```python
from build123d import *

# Parameters (mm, degrees)
F0_W     = 10
F0_H     = 25.0418604054
F0_H_2   = 18
F0_H_3   = 6.9581395946
F3_R     = 10
F4_DEPTH = 141.6
F7_D     = 3
F8_D     = 3
F9_R     = 2.99999


# Not quite as in the source:
# - a fillet or chamfer that OpenCascade refuses, or shapes differently, is made with other operations: its cross-section is extruded or revolved along the edge and cut away or added
# - a fillet or chamfer is up to 0.001 mm smaller than in the source, because OpenCascade refuses the exact size


with BuildPart() as f1:
    # F0 (on Front) → F1 (revolve)
    with BuildSketch(Plane.XZ):
        Polygon((-55, 15), (-55, 0), (0, 0), (0, 18), (-40, 18), (-40, 15), align=None)
    revolve(axis=Axis((0, 0, 9), (0, 0, 1)))

    # F0 (on Front) → F2 (revolve, cut)
    with BuildSketch(Plane.XZ):
        with Locations((5, 30.5209302027)):
            Rectangle(F0_W, F0_H)
        with Locations((5, 9)):
            Rectangle(F0_W, F0_H_2)
        with Locations((5, -3.4790697973)):
            Rectangle(F0_W, F0_H_3)
    revolve(axis=Axis((0, 0, 18.0418604054), (0, 0, 1)), mode=Mode.SUBTRACT)

    # F3 (on Front) → F4 (cut)
    with BuildSketch(Plane.XZ):
        Circle(F3_R)
    extrude(amount=-F4_DEPTH, mode=Mode.SUBTRACT)

    # F5: fillet of radius 15 on 1 edges, made by hand

    # F5_s1 → F5_t2 (revolve, cut)
    with BuildSketch(Plane.XZ):
        with BuildLine():
            ThreePointArc((-55, 0), (-50.6066017178, 10.6066017178), (-40, 15))
            Line((-40, 15), (-55, 15))
            Line((-55, 15), (-55, 0))
        make_face()
    revolve(axis=Axis((0, 0, 15), (0, 0, 1)), mode=Mode.SUBTRACT)

    # F7 (through all)
    with Locations(Plane(origin=(0, 0, 0), x_dir=(1, 0, 0), z_dir=(0, 0, -1))):
        with Locations((24, 0)):
            Hole(F7_D / 2)

    # F8 (through all)
    with Locations(Plane(origin=(0, 0, 0), x_dir=(1, 0, 0), z_dir=(0, 0, -1))):
        with Locations((-24, 0)):
            Hole(F8_D / 2)

    # F9 (radius 3 in the source; OpenCascade refuses exactly that, so slightly less here)
    f9_edges = [f1.edges().sort_by_distance(p)[0] for p in [
        (40, 0, 18),
    ]]
    fillet(f9_edges, radius=F9_R)


solid = f1.part
```
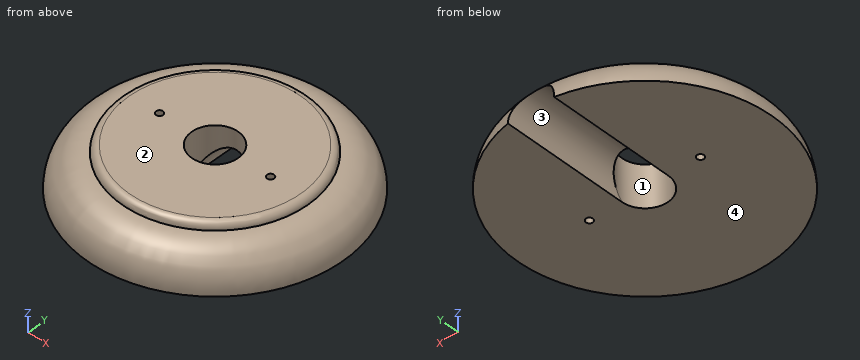
Here's how the part is built. I have some questions about the finished solid (model axes, mm). Face numbers are marked on the shaded views. A direction names the side the tool comes from. Coordinates: 2 decimals unless noted, no trailing zeros. Order: outer loops, then holes, each group sorted by start corner. A loop starts at its lowest first (then second) coordinate and runs counter-clockwise, first axis right, second up. Notation, with made-up numbers: (69, 79) - (89, 79) arc R36 cw to (89, 117) - close; hole circle Ø4 at (71.5, 55.5). An arc over 180 degrees is marked (long way). One line per question, with ' | ' between items.
(1) Suppose I cut it at B-B on z = 16.25. List the corners of the cut face in (x, y) for me, and give its area (3 significant figures).
Report:
outline: circle Ø79.45 at (0, 0); hole circle Ø3 at (-24, 0); hole circle Ø20 at (0, 0); hole circle Ø3 at (24, 0) | area: 4,630 mm2
(2) If we mould it in two halves opening along Y, with no side actions, what happens to the marked faces 1 and 2? For each: pulls with the +Y half, pulls with the -Y half, needs draft (parallel to the pull), parting line crosses it, or undercut.
Report:
face 1: undercut | face 2: needs draft
(3) If I drill on L1, parallel to Y at x = 23.5, z = 2; L2, parallel to X at y = 17.5, z = 5; L3, parallel to Y at x = 24, z = 13.5, over which ranges is the centre line in solid material (lowest first)?
Report:
L1: y = -49.58 to -1.41, 1.41 to 49.58 | L2: x = -51.24 to -8.66, 8.66 to 51.24 | L3: y = -39.87 to -1.5, 1.5 to 39.87
(4) Suppose I cut it at A-A on z = 8. List the corners of the cut face in (x, y) for me, and give its area (3 significant figures).
Report:
outline: (-6, 8) - (-6, 52.35) arc R52.69 ccw (long way) to (6, 52.35) - (6, 8) arc R10 cw (long way) to start; hole circle Ø3 at (-24, 0); hole circle Ø3 at (24, 0) | area: 7,870 mm2
(5) Will these pins go through, and if not, where does the flat tip stop? pin 1 (1.5 mm diameter, centred on x = 31, y = -22.5, fed in from +Z); pin 2 (3 mm diameter, centred on y = -7.5, z = 11.5, fed in from +X); pin 3 (1.5 mm diameter, centred on x = -34.5, z = 12, fed in from +Y).
Report:
pin 1: stops at z = 17.95 | pin 2: stops at x = 50.65 | pin 3: stops at y = 36.28
(6) For the marked faces 3 and 4, which set-ups out of +Z, -Z, +X, -X, +Y, -Y let a thin tool reach every point of the face, with its end or its side?
Report:
face 3: -Z, +Y | face 4: -Z, +X, -X, +Y, -Y
